from build123d import *

# Parameters (mm, degrees)
BODY_2_W                        = 35
BODY_2_H                        = 9
BODY_DEPTH                      = 5.5
HOLES_2_R                       = 0.6
HOLES_DEPTH                     = 1
CHANNEL_2_W                     = 28
CHANNEL_2_H                     = 2.5
CHANNEL_DEPTH                   = 0.5
CONNECTION_PINS_2_W             = 1.5
CONNECTION_PINS_2_H             = 0.4
CONNECTION_PINS_2_W_2           = 0.4
CONNECTION_PINS_2_H_2           = 1
CONNECTION_PINS_DEPTH           = 5
SKIZZE1_R                       = 0.25
SCHNITT_LINEAR_AUSTRAGEN1_DEPTH = 11


with BuildPart() as part:
    # body 2 → body (new body)
    with BuildSketch(Plane.XY):
        Rectangle(BODY_2_W, BODY_2_H)
    extrude(amount=BODY_DEPTH)

    # holes 2 → holes (cut)
    with BuildSketch(Plane.XY.offset(5.5)):
        with Locations((-15.5, 0)):
            Circle(HOLES_2_R)
        with Locations((15.5, 0)):
            Circle(HOLES_2_R)
    extrude(amount=-HOLES_DEPTH, mode=Mode.SUBTRACT)

    # channel 2 → channel (cut)
    with BuildSketch(Plane.XY.offset(5.5)):
        Rectangle(CHANNEL_2_W, CHANNEL_2_H)
    extrude(amount=-CHANNEL_DEPTH, mode=Mode.SUBTRACT)

    # connection pins 2 → connection pins (add)
    with BuildSketch(Plane(origin=(0, 0, 0), x_dir=(-1, 0, 0), z_dir=(0, 0, -1))):
        with Locations((-12.6, 4.3)):
            Rectangle(CONNECTION_PINS_2_W, CONNECTION_PINS_2_H)
        with Locations((12.6, 4.3)):
            Rectangle(CONNECTION_PINS_2_W, CONNECTION_PINS_2_H)
        with Locations((-11.4, -4.3)):
            Rectangle(CONNECTION_PINS_2_W, CONNECTION_PINS_2_H)
        with Locations((-17.3, -1.75)):
            Rectangle(CONNECTION_PINS_2_W_2, CONNECTION_PINS_2_H_2)
        with Locations((11.4, -4.3)):
            Rectangle(CONNECTION_PINS_2_W, CONNECTION_PINS_2_H)
        with Locations((17.3, 1.75)):
            Rectangle(CONNECTION_PINS_2_W_2, CONNECTION_PINS_2_H_2)
        with Locations((17.3, -1.75)):
            Rectangle(CONNECTION_PINS_2_W_2, CONNECTION_PINS_2_H_2)
    extrude(amount=CONNECTION_PINS_DEPTH)

    # Skizze1 → Schnitt-Linear austragen1 (cut, through all)
    with BuildSketch(Plane.XY.offset(5)):
        Circle(SKIZZE1_R)
    extrude(amount=-SCHNITT_LINEAR_AUSTRAGEN1_DEPTH, mode=Mode.SUBTRACT)


solid = part.part
For this review, take the finished solid that the model builds, in its own axes (mm). A direction names the side the tool comes from. Round coordinates to 2 decimals unless told otherwise and drop trailing zeros. Write each loop counter-clockwise with the first axis right and the second up, starting at its lowest first coordinate (ties: lowest second). Pieces come first, ordered by that corner, then holes. Notation, with made-up numbers: (54.25, -5) -> (95.25, -5) arc R17 cw to (95.25, 2) -> close; hole circle Ø4 at (68, 1.25). An arc over 180 degrees is marked (long way). Put each result on its own line as item: value.
Q1. Clearance check with a flat-ended pin moving along its axis: pin 1 Ø4.5 at (x, y) = (-4.5, 1.5) entering from -Z. State where the tip first meets the part, or that it passes through.
Determined:
pin 1: stops at z = 0
Q2. Consider section A-A on x = 4. State the section outline as (y, z) points, and give its area (4 significant figures).
Determined:
outline: (-4.5, 0) -> (4.5, 0) -> (4.5, 5.5) -> (1.25, 5.5) -> (1.25, 5) -> (-1.25, 5) -> (-1.25, 5.5) -> (-4.5, 5.5) -> close
area: 48.25 mm^2
Q3. The part is to be moulded in two halves that separate along Y. For faces 1 (the flat face through (0, 1, 5)), 2 (the flat face through (0, 2, 5.5)), 3 (the flat face through (0, 4.5, 3)), say which applies: released by +Y, released by -Y, zero draft, split by the parting line, or undercut.
Determined:
face 1: undercut
face 2: zero draft
face 3: released by +Y
Q4. Consider section B-B on y = -3.5. State the section outline as (x, z) points, and give its area (4 significant figures).
Determined:
outline: (-17.5, 0) -> (17.5, 0) -> (17.5, 5.5) -> (-17.5, 5.5) -> close
area: 192.5 mm^2
Q5. To check wall thickness, follow L1, parallel to Y at x = -15.5, z = 5; L2, parallel to Y at x = 0, z = 0.25; L3, parallel to Z at x = 12.5, y = 4. State the ranges of each line that lie inside material, in increasing order. Write a range as [from, to].
Determined:
L1: y = [-4.5, -0.6], [0.6, 4.5]
L2: y = [-4.5, -0.25], [0.25, 4.5]
L3: z = [0, 5.5]
Q6. Consider section C-C on x = -15.5. State the section outline as (y, z) points, and give its area (3 significant figures).
Determined:
outline: (-4.5, 0) -> (4.5, 0) -> (4.5, 5.5) -> (0.6, 5.5) -> (0.6, 4.5) -> (-0.6, 4.5) -> (-0.6, 5.5) -> (-4.5, 5.5) -> close
area: 48.3 mm^2
Q7. Machinability: for faces 4 (the flat face through (13, 4.1, -2)), 5 (the cylindrical face through (-14.946, -0.23, 5.007)), 6 (the flat face through (17.1, -2, -2)), 7 (the flat face through (-17.5, 0, 1)), 8 (the flat face through (-17.1, 2, -2)), which of the approach directions +Z, -Z, +X, -X, +Y, -Y give a long, thin tool a straight path to every point of the face, cutting with its end or side? Answer none if there is none.
Determined:
face 4: -Z, +X, -X
face 5: +Z
face 6: -Z, +Y, -Y
face 7: +Z, -Z, -X, +Y, -Y
face 8: -Z, +X, +Y, -Y
